Answer from the drawing. Dimensions are ordinates in mm from the lowest x, y and z of the part. Coordinates: 2 decimals unless noted, no trailing zeros. Order: outer loops, then holes, each group sorted by start corner. A loop starts at its lowest first (then second) coordinate and runs counter-clockwise, first axis right, second up. Notation, with made-up numbers: (39.25, 7.5) -> (71.25, 7.5) arc R20 cw to (71.25, 15.5) -> close; hole circle Ø4 at (66, 66). An arc over 180 degrees is marked (long way). Use CSV: the item, a comma, the result in double quotes.
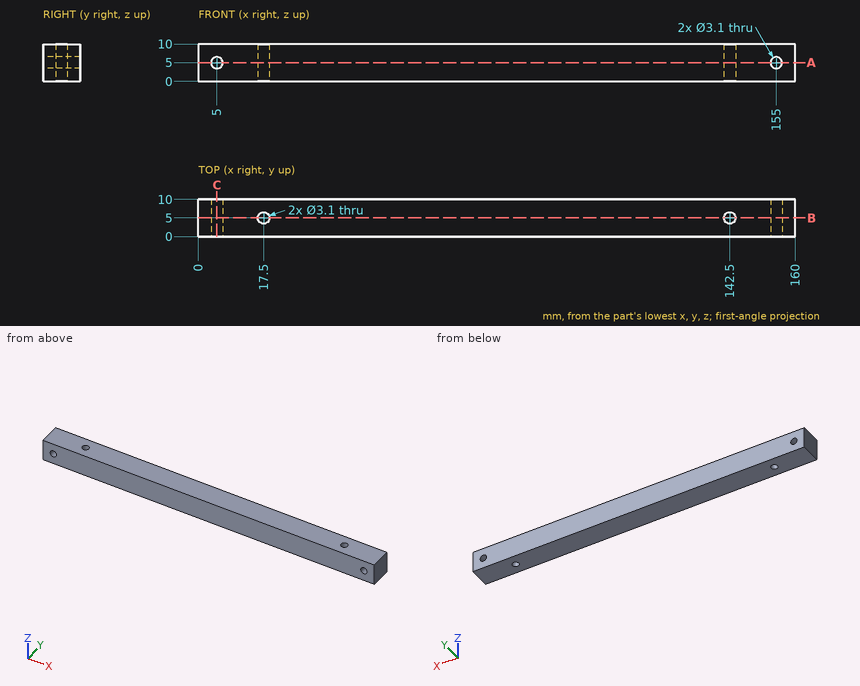
Item 1: Find section C-C, the plane x = 5. Give the vertices of the cut face in (y, z).
Return value:
outline,"(0, 0) -> (10, 0) -> (10, 3.45) -> (0, 3.45) -> close; (0, 6.55) -> (10, 6.55) -> (10, 10) -> (0, 10) -> close"
Item 2: Find section A-A, the plane z = 5. Give the vertices of the cut face in (x, y).
Return value:
outline,"(0, 0) -> (3.45, 0) -> (3.45, 10) -> (0, 10) -> close; (6.55, 0) -> (153.45, 0) -> (153.45, 10) -> (6.55, 10) -> close; (156.55, 0) -> (160, 0) -> (160, 10) -> (156.55, 10) -> close; hole circle Ø3.1 at (17.5, 5); hole circle Ø3.1 at (142.5, 5)"
Item 3: Find section B-B, the plane y = 5. Give the vertices of the cut face in (x, z), then the cut area to 3 significant figures.
Return value:
outline,"(0, 0) -> (15.95, 0) -> (15.95, 10) -> (0, 10) -> close; (19.05, 0) -> (140.95, 0) -> (140.95, 10) -> (19.05, 10) -> close; (144.05, 0) -> (160, 0) -> (160, 10) -> (144.05, 10) -> close; hole circle Ø3.1 at (5, 5); hole circle Ø3.1 at (155, 5)"
area,"1,520 mm^2"
Item 4: Straight lines are drawn through the part: line 1 along X through (y, z) = (3, 5); line 2 along Y through (x, z) = (142.5, 2.5); line 3 along X through (y, z) = (4.75, 0.5). For each, find the intervals that lie inside material, in ascending order.
Return value:
line 1,"x = 0 to 3.45, 6.55 to 153.45, 156.55 to 160"
line 2,"y = 0 to 3.45, 6.55 to 10"
line 3,"x = 0 to 15.97, 19.03 to 140.97, 144.03 to 160"
